Read the model definition and answer for the solid it produces. Units are mm, in the model's axes. Face numbers are marked on the shaded views. Give positions to 0.01 mm unless a question says otherwise; leave off trailing zeros. Loops run counter-clockwise (first coordinate to the right, second up) from the corner with the lowest first, then second, coordinate; pieces in that order, holes last. Notation, with made-up numbers: (24.5, -21.75) -> (61.5, -21.75) arc R20 ccw to (61.5, -14.75) -> close; hole circle Ø9 at (17.25, -23.75). An arc over 180 degrees is marked (long way). One line per item, written item: value. Start each with the question number.
Solid Edge part; units mm, degrees
sketch "Sketch1" plane through (0, 0, 0) normal (0, 0, 1) x (1, 0, 0)
  line L0 (30, 75) -> (30, 30)
  line L1 (30, 30) -> (60, 30)
  line L2 (60, 30) -> (60, 75)
  line L3 (60, 75) -> (30, 75)
  line L4 (120, 30) -> (0, 30)
  line L5 (0, 30) -> (0, 0)
  line L6 (0, 0) -> (120, 0)
  line L7 (120, 0) -> (120, 30)
extrude "Protrusion1" add sketch "Sketch1" along normal blind 4
fillet "RoundMain" radius 15 6 edges at (0, 30, 2) (30, 75, 2) (60, 75, 2) (120, 30, 2) (120, 0, 2) (0, 0, 2)
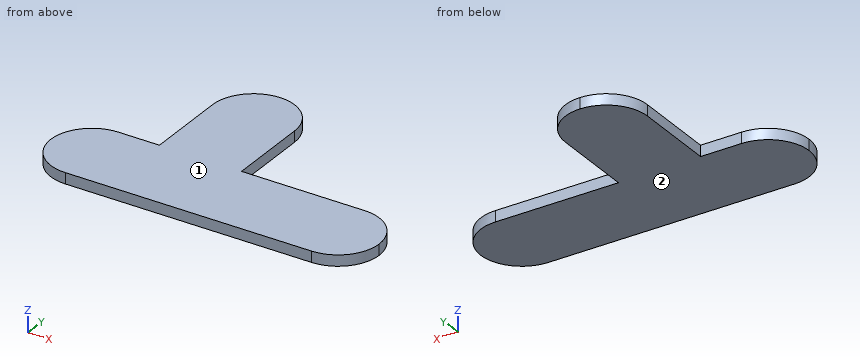
Item 1: Section C-C, the plane x = 87.5 is taken. Determine the outline of the cut face in (y, z).
Item 2: Section B-B, the plane y = 48.5 is taken. Determine the outline of the cut face in (x, z).
Item 3: Consider L1, parallel to X at y = 57, z = 0.45; L2, parallel to Y at x = 22, z = 2.15; L3, parallel to Y at x = 44.5, z = 0.3. Determine where each line is inside the solid, lowest interval first. Write a range as [from, to].
Item 4: Flat-ended cylindrical pins translate along their axes: pin 1 (2 mm diameter, centred on y = 10.5, z = 3.5, fed in from +X); pin 2 (2 mm diameter, centred on x = 95.5, z = 1.5, fed in from +Y); pin 3 (1 mm diameter, centred on x = 52, z = 3, fed in from -Y). Find the tip coordinate at first contact, or state that the pin passes through.
Item 5: Determine the mould class of the marked faces 1 and 2 for opening direction Z: pulls with the +Z half, pulls with the -Z half, needs draft (parallel to the pull), parting line crosses it, or undercut.
Computed values:
1. outline: (0, 0) -> (30, 0) -> (30, 4) -> (0, 4) -> close
2. outline: (30, 0) -> (60, 0) -> (60, 4) -> (30, 4) -> close
3. L1: [30, 60]
3. L2: [0, 30]
3. L3: [0, 74.99]
4. pin 1: x = 119.59
4. pin 2: y = 30
4. pin 3: y = 0
5. face 1: pulls with the +Z half
5. face 2: pulls with the -Z half
